```python
from build123d import *

# Parameters (mm, degrees)
SKETCH1_W               = 50.8
SKETCH1_H               = 25.4
BOSS_EXTRUDE1_DEPTH     = 381
SHELL1_T                = -3.175
CUT_EXTRUDE2_DEPTH      = 383.689587002
CUT_EXTRUDE2_DEPTH_BACK = 383.689587002
SKETCH5_R               = 2.38125


with BuildPart() as part:
    # Sketch1 → Boss-Extrude1 (new, symmetric)
    with BuildSketch(Plane(origin=(0, 0, 0), x_dir=(1, 0, 0), z_dir=(0, 1, 0))):
        Rectangle(SKETCH1_W, SKETCH1_H)
    extrude(amount=BOSS_EXTRUDE1_DEPTH, both=True)

    # Shell1
    shell1_openings = [part.faces().sort_by_distance(p)[0] for p in [
        (0, 381, 0),
        (0, -381, 0),
    ]]
    offset(amount=SHELL1_T, openings=shell1_openings, kind=Kind.INTERSECTION)

    # Sketch5 → Cut-Extrude2 (cut, two sides: drawn at the far end of the back side and taken through both)
    with BuildSketch(Plane.XY.offset(12.7).offset(-CUT_EXTRUDE2_DEPTH_BACK)):
        with Locations((-12.7, 368.3)):
            Circle(SKETCH5_R)
        with Locations((12.7, 368.3)):
            Circle(SKETCH5_R)
        with Locations((12.7, 342.9)):
            Circle(SKETCH5_R)
        with Locations((-12.7, 342.9)):
            Circle(SKETCH5_R)
        with Locations((-12.7, -342.9)):
            Circle(SKETCH5_R)
        with Locations((12.7, -342.9)):
            Circle(SKETCH5_R)
        with Locations((12.7, -368.3)):
            Circle(SKETCH5_R)
        with Locations((-12.7, -368.3)):
            Circle(SKETCH5_R)
        with Locations((-12.7, 12.7)):
            Circle(SKETCH5_R)
        with Locations((12.7, 12.7)):
            Circle(SKETCH5_R)
        with Locations((12.7, -12.7)):
            Circle(SKETCH5_R)
        with Locations((-12.7, -12.7)):
            Circle(SKETCH5_R)
        with Locations((-12.7, 317.5)):
            Circle(SKETCH5_R)
        with Locations((12.7, 317.5)):
            Circle(SKETCH5_R)
        with Locations((12.7, 292.1)):
            Circle(SKETCH5_R)
        with Locations((-12.7, 292.1)):
            Circle(SKETCH5_R)
        with Locations((-12.7, -292.1)):
            Circle(SKETCH5_R)
        with Locations((12.7, -292.1)):
            Circle(SKETCH5_R)
        with Locations((12.7, -317.5)):
            Circle(SKETCH5_R)
        with Locations((-12.7, -317.5)):
            Circle(SKETCH5_R)
    extrude(amount=CUT_EXTRUDE2_DEPTH + CUT_EXTRUDE2_DEPTH_BACK, mode=Mode.SUBTRACT)


solid = part.part
```
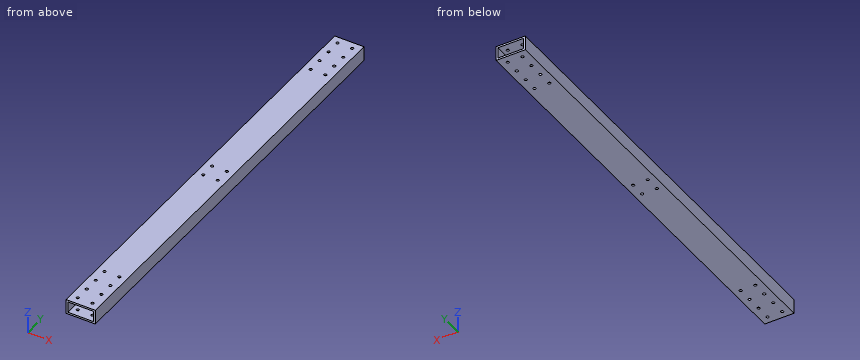
Can you work these out from the model? Positions are in its coordinate system, mm. Give positions to 0.01 mm unless a question says otherwise; leave off trailing zeros. Write each loop counter-clockwise with the first axis right and the second up, starting at its lowest first coordinate (ties: lowest second). Pieces come first, ordered by that corner, then holes. Notation, with made-up numbers: (-24, 14) - (11, 14) arc R15 ccw to (11, 37) - close; hole circle Ø4 at (4.5, -3). An arc over 180 degrees is marked (long way). Write item = value, one per line. Start each with the question number.
1. Imagine slicing it at A-A (z = -2). Please give me the cut outline in (x, y) (3 decimals), and give its area (3 significant figures).
2. Please list where these lines run through material, in increasing order: line 1 (X direction, y = -12.7, z = -11.6); line 2 (Z direction, x = 0, y = 107) (3 decimals); line 3 (X direction, y = 102.5, z = 0.25) (3 decimals).
3. Imagine slicing it at C-C (x = -3.5). Please give me the cut outline in (y, z) (3 decimals), and give its area (3 significant figures).
4. For pin 1 (7.5 mm diameter, centred on x = 12.7, y = -12.7, fed in from -Z), with a flat end and sliding along its axis, tell me the tip position at first contact or that it passes through.
5. Imagine slicing it at B-B (y = -271). Please give me the cut outline in (x, z) (3 decimals), and give its area (3 significant figures).
Worked answers:
q1.outline = (-25.4, -381) - (-22.225, -381) - (-22.225, 381) - (-25.4, 381) - close; (22.225, -381) - (25.4, -381) - (25.4, 381) - (22.225, 381) - close
q1.area = 4,840 mm2
q2.line_1 = -25.4 to -15.08, -10.32 to 10.32, 15.08 to 25.4
q2.line_2 = -12.7 to -9.525, 9.525 to 12.7
q2.line_3 = -25.4 to -22.225, 22.225 to 25.4
q3.outline = (-381, -12.7) - (381, -12.7) - (381, -9.525) - (-381, -9.525) - close; (-381, 9.525) - (381, 9.525) - (381, 12.7) - (-381, 12.7) - close
q3.area = 4,840 mm2
q4.pin_1 = -12.7
q5.outline = (-25.4, -12.7) - (25.4, -12.7) - (25.4, 12.7) - (-25.4, 12.7) - close; hole (-22.225, -9.525) - (22.225, -9.525) - (22.225, 9.525) - (-22.225, 9.525) - close
q5.area = 444 mm2
